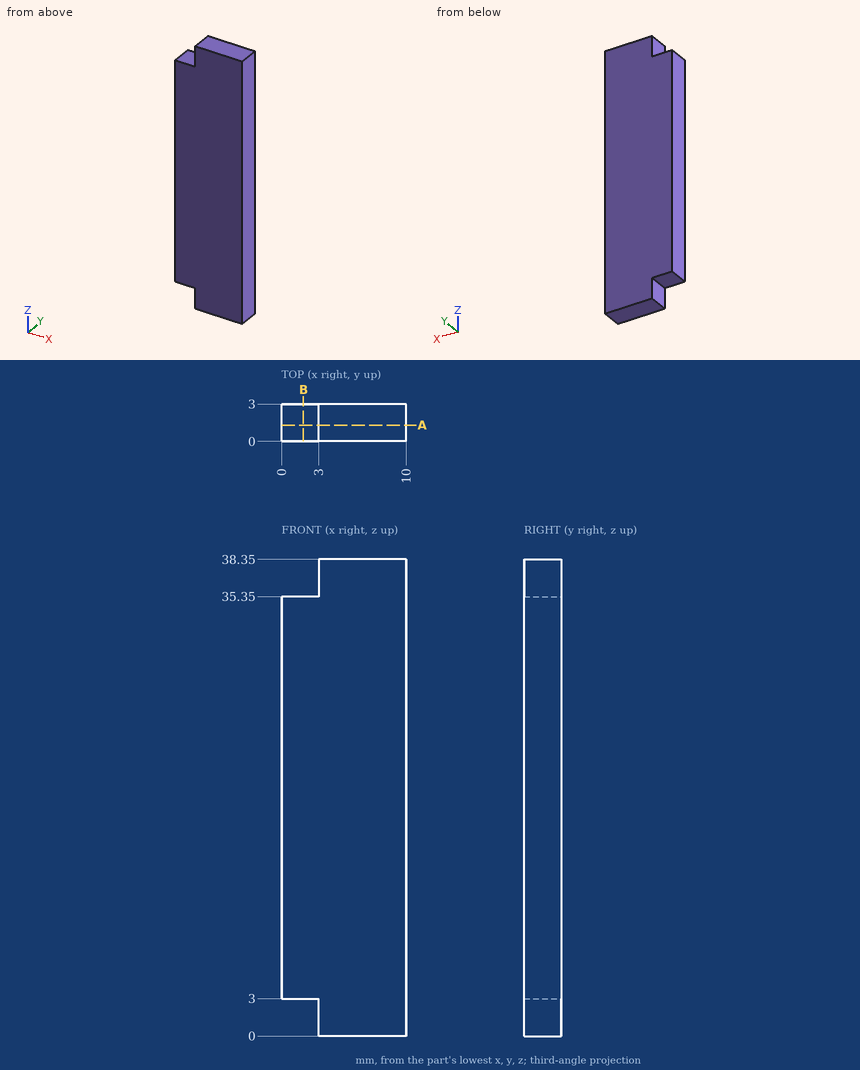
Study the drawing (mm; zero at the part's minimum x, y, z) and answer. Round coordinates to 2 decimals unless told otherwise and drop trailing zeros. Write each loop counter-clockwise with the first axis right and the second up, starting at its lowest first coordinate (ties: lowest second). Pieces come first, ordered by that corner, then holes. Notation, with made-up numbers: (61, 58) -> (75, 58) arc R22 cw to (75, 83) -> close; hole circle Ø3 at (38, -27). An arc over 180 degrees is marked (long way). Write item = value, one per line.
1) Section B-B on x = 1.75 is taken. Write down the section's boundary in (y, z).
Check values:
outline = (0, 3) -> (3, 3) -> (3, 35.35) -> (0, 35.35) -> close
2) Given pin 1 (1.5 mm diameter, centred on x = 2, y = 1, fed in from -Z); pin 2 (1.5 mm diameter, centred on x = 1, y = 2, fed in from +Z); pin 3 (1.5 mm diameter, centred on y = 1.5, z = 36.5, fed in from -X), each flat-ended and moving along its own axis, determine where each tip first touches the part or whether it passes through.
Check values:
pin_1 = 3
pin_2 = 35.35
pin_3 = 3
3) Straight lines are drawn through the part: line 1 along X through (y, z) = (2.7, 2); line 2 along Z through (x, y) = (1.75, 0.6). For each, find the intervals that lie inside material, in ascending order. Write a range as [from, to].
Check values:
line_1 = [3, 10]
line_2 = [3, 35.35]
4) Section A-A on y = 1.3 is taken. Write down the section's boundary in (x, z), plus the area to 4 significant figures.
Check values:
outline = (0, 3) -> (3, 3) -> (3, 0) -> (10, 0) -> (10, 38.35) -> (3, 38.35) -> (3, 35.35) -> (0, 35.35) -> close
area = 365.5 mm²
